Source: three-view drawing plus pictorial views. Frame: mm from the lowest corner of the part. A direction names the side the tool comes from. Coordinates: 2 decimals unless noted, no trailing zeros. Order: outer loops, then holes, each group sorted by start corner. A loop starts at its lowest first (then second) coordinate and runs counter-clockwise, first axis right, second up. Notation, with made-up numbers: (60.25, -40) -> (99.25, -40) arc R24 cw to (99.25, -18) -> close; hole circle Ø4 at (27.25, 9). An arc over 180 degrees is marked (long way). Use CSV: the item, a comma, the result in double quotes. Start each with the question number.
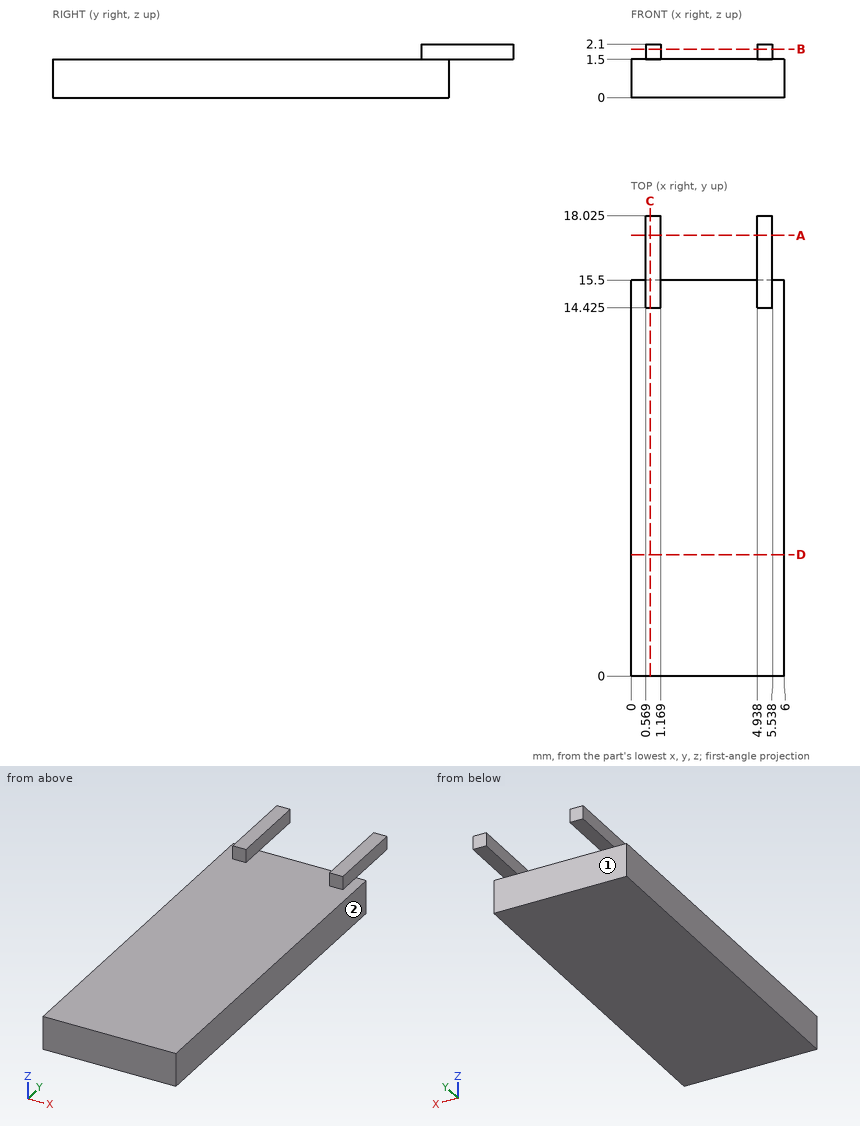
1. Material intervals for line 1 along Y through (x, z) = (2.9, 0.2); line 2 along Z through (x, y) = (4.85, 13), sorted ascending.
2. Access query for the marked faces 1 and 2. Directions: +Z, -Z, +X, -X, +Y, -Y. A direction counts if a zero-diameter tool reaches every point of the face in a straight line with its end or side. Return the directions, or none.
3. Section B-B on z = 1.9. Return loops of the section in (x, y) (1 decimal).
4. Section C-C on x = 0.75. Return loops of the section in (y, z) (1 decimal), then the cut area to 3 significant figures.
5. Section D-D on y = 4.75. Return loops of the section in (x, z).
6. Contact query for flat-ended pins moving along their axis: P1, Ø0.7, axis at x = 1, y = 17, coming from the -Z side; P2, Ø0.7, axis at x = 5, z = 2, coming from the -Y side (3 decimals); P3, Ø1.2, axis at x = 4, z = 1, coming from the +Y side. Output: stop coordinate, or through.
7. Section A-A on y = 17.25. Return loops of the section in (x, z).
Values follow:
1,line 1,"y = 0 to 15.5"
1,line 2,"z = 0 to 1.5"
2,face 1,"-Z, +X, -X, +Y"
2,face 2,"+Z, -Z, +X, +Y, -Y"
3,outline,"(0.6, 14.4) -> (1.2, 14.4) -> (1.2, 18) -> (0.6, 18) -> close; (4.9, 14.4) -> (5.5, 14.4) -> (5.5, 18) -> (4.9, 18) -> close"
4,outline,"(0, 0) -> (15.5, 0) -> (15.5, 1.5) -> (18, 1.5) -> (18, 2.1) -> (14.4, 2.1) -> (14.4, 1.5) -> (0, 1.5) -> close"
4,area,"25.4 mm2"
5,outline,"(0, 0) -> (6, 0) -> (6, 1.5) -> (0, 1.5) -> close"
6,P1,"stops at z = 1.5"
6,P2,"stops at y = 14.425"
6,P3,"stops at y = 15.5"
7,outline,"(0.57, 1.5) -> (1.17, 1.5) -> (1.17, 2.1) -> (0.57, 2.1) -> close; (4.94, 1.5) -> (5.54, 1.5) -> (5.54, 2.1) -> (4.94, 2.1) -> close"
